The model under review builds one solid part; all positions refer to its coordinate system, in mm. Face numbers are marked on the shaded views. A direction names the side the tool comes from. Coordinates: 2 decimals unless noted, no trailing zeros. Write each loop counter-clockwise with the first axis right and the second up, starting at its lowest first coordinate (ties: lowest second). Pieces come first, ordered by that corner, then holes.
```python
from build123d import *

# Parameters (mm, degrees)
F1_DEPTH = 40
F2_DEPTH = 32.5
F3_DEPTH = 25


with BuildPart() as f1:
    # F0 (on Top) → F1 (new body, symmetric)
    with BuildSketch(Plane.XY):
        with BuildLine():
            Line((0, 7.5), (0, 15))
            ThreePointArc((0, 15), (-10.606602, 10.606602), (-15, 0))
            Line((-15, 0), (-7.5, 0))
            ThreePointArc((-7.5, 0), (-5.303301, 5.303301), (0, 7.5))
        make_face()
        with BuildLine():
            ThreePointArc((0, -15), (10.606602, -10.606602), (15, 0))
            Line((15, 0), (7.5, 0))
            ThreePointArc((7.5, 0), (5.303301, -5.303301), (0, -7.5))
            Line((0, -7.5), (0, -15))
        make_face()
        with BuildLine():
            ThreePointArc((0, -7.5), (5.303301, -5.303301), (7.5, 0))
            ThreePointArc((7.5, 0), (5.303301, 5.303301), (0, 7.5))
            ThreePointArc((0, 7.5), (-5.303301, 5.303301), (-7.5, 0))
            ThreePointArc((-7.5, 0), (-5.303301, -5.303301), (0, -7.5))
        make_face()
    extrude(amount=F1_DEPTH, both=True)

    # F0 (on Top) → F2 (cut, symmetric)
    with BuildSketch(Plane.XY):
        with BuildLine():
            Line((0, 7.5), (0, 15))
            ThreePointArc((0, 15), (-10.606602, 10.606602), (-15, 0))
            Line((-15, 0), (-7.5, 0))
            ThreePointArc((-7.5, 0), (-5.303301, 5.303301), (0, 7.5))
        make_face()
        with BuildLine():
            ThreePointArc((0, -15), (10.606602, -10.606602), (15, 0))
            Line((15, 0), (7.5, 0))
            ThreePointArc((7.5, 0), (5.303301, -5.303301), (0, -7.5))
            Line((0, -7.5), (0, -15))
        make_face()
    extrude(amount=F2_DEPTH, both=True, mode=Mode.SUBTRACT)

    # F0 (on Top) → F3 (join, symmetric)
    with BuildSketch(Plane.XY):
        with BuildLine():
            Line((0, 7.5), (0, 15))
            ThreePointArc((0, 15), (-10.606602, 10.606602), (-15, 0))
            Line((-15, 0), (-7.5, 0))
            ThreePointArc((-7.5, 0), (-5.303301, 5.303301), (0, 7.5))
        make_face()
        with BuildLine():
            ThreePointArc((-15, 0), (-10.606602, -10.606602), (0, -15))
            Line((0, -15), (0, -7.5))
            ThreePointArc((0, -7.5), (-5.303301, -5.303301), (-7.5, 0))
            Line((-7.5, 0), (-15, 0))
        make_face()
        with BuildLine():
            Line((7.5, 0), (15, 0))
            ThreePointArc((15, 0), (10.606602, 10.606602), (0, 15))
            Line((0, 15), (0, 7.5))
            ThreePointArc((0, 7.5), (5.303301, 5.303301), (7.5, 0))
        make_face()
        with BuildLine():
            ThreePointArc((0, -15), (10.606602, -10.606602), (15, 0))
            Line((15, 0), (7.5, 0))
            ThreePointArc((7.5, 0), (5.303301, -5.303301), (0, -7.5))
            Line((0, -7.5), (0, -15))
        make_face()
    extrude(amount=F3_DEPTH, both=True)


solid = f1.part
```
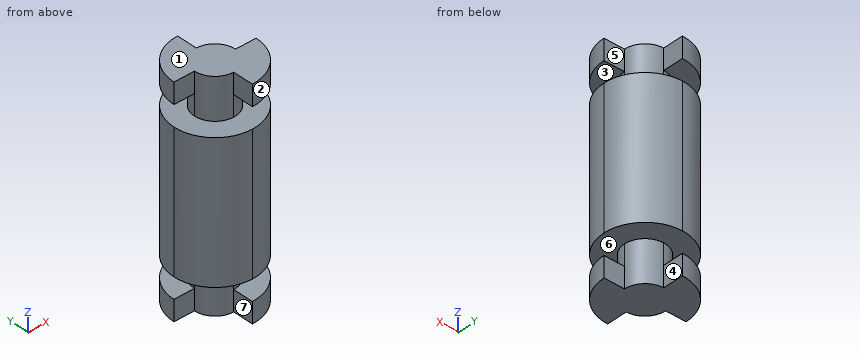
Item 1: Mouldability with a two-part tool opening along Z and no side actions: class the marked faces 1, 2 and 3 as pulls with the +Z half, pulls with the -Z half, needs draft (parallel to the pull), parting line crosses it, or undercut.
Solved:
face 1: pulls with the +Z half
face 2: needs draft
face 3: undercut
Item 2: For pin 1 (4 mm diameter, centred on y = 8.5, z = -24.5, fed in from -X); pin 2 (4 mm diameter, centred on y = 11.5, z = -36.5, fed in from +X); pin 3 (6 mm diameter, centred on y = -11.5, z = 36.5, fed in from -X), all flat-tipped, find the tip position at first contact; note any pin that passes through.
Solved:
pin 1: stops at x = -13.52
pin 2: stops at x = 0
pin 3: stops at x = 0
Item 3: Take a section at B-B, the plane x = 12.5. Write out the cut boundary in (y, z).
Solved:
outline: (-8.29, -40) - (0, -40) - (0, -32.5) - (-8.29, -32.5) - close; (-8.29, -25) - (8.29, -25) - (8.29, 25) - (-8.29, 25) - close; (-8.29, 32.5) - (0, 32.5) - (0, 40) - (-8.29, 40) - close
Item 4: Take a section at C-C, the plane x = 6.5. Write out the cut boundary in (y, z).
Solved:
outline: (-13.52, -40) - (3.74, -40) - (3.74, -25) - (13.52, -25) - (13.52, 25) - (3.74, 25) - (3.74, 40) - (-13.52, 40) - (-13.52, 32.5) - (-3.74, 32.5) - (-3.74, 25) - (-13.52, 25) - (-13.52, -25) - (-3.74, -25) - (-3.74, -32.5) - (-13.52, -32.5) - close
Item 5: Take a section at A-A, the plane y = 13. Write out the cut boundary in (x, z).
Solved:
outline: (-7.48, -40) - (0, -40) - (0, -32.5) - (-7.48, -32.5) - close; (-7.48, -25) - (7.48, -25) - (7.48, 25) - (-7.48, 25) - close; (-7.48, 32.5) - (0, 32.5) - (0, 40) - (-7.48, 40) - close
Item 6: Take a section at D-D, the plane y = -1.5. Write out the cut boundary in (x, z).
Solved:
outline: (-14.92, -25) - (-7.35, -25) - (-7.35, -40) - (14.92, -40) - (14.92, -32.5) - (7.35, -32.5) - (7.35, -25) - (14.92, -25) - (14.92, 25) - (7.35, 25) - (7.35, 32.5) - (14.92, 32.5) - (14.92, 40) - (-7.35, 40) - (-7.35, 25) - (-14.92, 25) - close
Item 7: Machinability: for the marked faces 4, 5, 6 and 7, which of the approach directions +Z, -Z, +X, -X, +Y, -Y give a long, thin tool a straight path to every point of the face, cutting with its end or side? Answer none if there is none.
Solved:
face 4: -Z, +X, +Y
face 5: +Z, +X, +Y
face 6: none
face 7: -Z, -X, -Y
Item 8: To check wall thickness, follow line 1 along Z through (x, y) = (6, -13); line 2 along Z through (x, y) = (7, 9); line 3 along X through (y, z) = (-7.5, -8). State the ranges of each line that lie inside material, in increasing order.
Solved:
line 1: z = -40 to -32.5, -25 to 25, 32.5 to 40
line 2: z = -25 to 25
line 3: x = -12.99 to 12.99
